```python
from build123d import *

# Parameters (mm, degrees)
ESQUISSE1_W             = 60
ESQUISSE1_H             = 60
ESQUISSE1_R             = 20
BOSS_EXTRU_1_DEPTH      = 25
CONG_1_R                = 1
TROU_TARAUD_M61_REACH   = 73.589
TROU_TARAUD_M61_BORE_R  = 2.5
TROU_TARAUD_M41_D       = 3.3
TROU_TARAUD_M41_DEPTH   = 7.5
TROU_TARAUD_M41_TIP     = 0.991420021
TROU_TARAUD_M42_D       = 3.3
TROU_TARAUD_M42_DEPTH   = 10.5
TROU_TARAUD_M42_TIP     = 0.991420021
ENL_V_MAT_EXTRU_1_REACH = 51.244
ENL_V_MAT_EXTRU_2_DEPTH = 3


with BuildPart() as part:
    # Esquisse1 → Boss.-Extru.1 (new body)
    with BuildSketch(Plane(origin=(0, 0, 0), x_dir=(1, 0, 0), z_dir=(0, 1, 0))):
        Rectangle(ESQUISSE1_W, ESQUISSE1_H)
        with Locations(Location((0, 0, 0), (0, 0, 270))):
            Circle(ESQUISSE1_R, mode=Mode.SUBTRACT)
    extrude(amount=BOSS_EXTRU_1_DEPTH)

    # Congé1
    cong_1_edges = [part.edges().sort_by_distance(p)[0] for p in [
        (30, 25, 0),
        (0, 25, -30),
        (-30, 25, 0),
        (0, 0, -30),
        (30, 0, 0),
        (0, 0, 30),
        (-30, 0, 0),
        (0, 25, 30),
        (-30, 12.5, -30),
        (30, 12.5, -30),
        (30, 12.5, 30),
        (-30, 12.5, 30),
    ]]
    fillet(cong_1_edges, radius=CONG_1_R)

    # Trou taraudé M61 bore → Trou taraudé M61 (cut, up to next)
    with BuildSketch(Plane.XY.offset(30), mode=Mode.PRIVATE) as trou_taraud_m61_sk1:
        with Locations((0, 12.5)):
            Circle(TROU_TARAUD_M61_BORE_R)
    trou_taraud_m61_tool1 = extrude(trou_taraud_m61_sk1.sketch, amount=-TROU_TARAUD_M61_REACH, mode=Mode.PRIVATE) & part.part
    add(trou_taraud_m61_tool1.solids().sort_by_distance((0, 12.5, 30))[0], mode=Mode.SUBTRACT)

    # Trou taraudé M41
    with Locations(Plane(origin=(0, 0, -30), x_dir=(-1, 0, 0), z_dir=(0, 0, -1))):
        with Locations((11.7, 12.5), (-11.7, 12.5)):
            Hole(TROU_TARAUD_M41_D / 2, depth=TROU_TARAUD_M41_DEPTH)
            with Locations((0, 0, -(TROU_TARAUD_M41_DEPTH + TROU_TARAUD_M41_TIP / 2))):  # 118° drill point
                Cone(0, TROU_TARAUD_M41_D / 2, TROU_TARAUD_M41_TIP, mode=Mode.SUBTRACT)

    # Trou taraudé M42
    with Locations(Plane.ZY.offset(30)):
        with Locations((-9.666666667, 12.5)):
            Hole(TROU_TARAUD_M42_D / 2, depth=TROU_TARAUD_M42_DEPTH)
            with Locations((0, 0, -(TROU_TARAUD_M42_DEPTH + TROU_TARAUD_M42_TIP / 2))):  # 118° drill point
                Cone(0, TROU_TARAUD_M42_D / 2, TROU_TARAUD_M42_TIP, mode=Mode.SUBTRACT)

    # Esquisse10 → Enlèv. mat.-Extru.1 (cut, up to next)
    with BuildSketch(Plane.XZ, mode=Mode.PRIVATE) as enl_v_mat_extru_1_sk1:
        with BuildLine():
            Line((-6, 19.078784028), (-6, 23.3))
            Line((-6, 23.3), (6, 23.3))
            Line((6, 23.3), (6, 19.078784028))
            ThreePointArc((6, 19.078784028), (0, 20), (-6, 19.078784028))
        make_face()
    enl_v_mat_extru_1_tool1 = extrude(enl_v_mat_extru_1_sk1.sketch, amount=-ENL_V_MAT_EXTRU_1_REACH, mode=Mode.PRIVATE) & part.part
    add(enl_v_mat_extru_1_tool1.solids().sort_by_distance((0, 0, 21.487514))[0], mode=Mode.SUBTRACT)

    # Esquisse11 → Enlèv. mat.-Extru.2 (cut)
    with BuildSketch(Plane.XZ):
        with BuildLine():
            Line((-10, 30), (-10, 17.320508076))
            ThreePointArc((-10, 17.320508076), (0, 20), (10, 17.320508076))
            Line((10, 17.320508076), (10, 30))
            Line((10, 30), (-10, 30))
        make_face()
    enl_v_mat_extru_2 = extrude(amount=-ENL_V_MAT_EXTRU_2_DEPTH, mode=Mode.SUBTRACT)

    # Esquisse13 → Trou taraudé M31 (revolve, cut)
    with BuildSketch(Plane(origin=(0, 3, 26), x_dir=(0, 0, -1), z_dir=(1, 0, 0))):
        Polygon((0, 0), (0, 6.251075774), (1.25, 5.5), (1.25, 0), align=None)
    trou_taraud_m31 = revolve(axis=Axis((0, -3.35, 26), (0, 1, 0)), mode=Mode.SUBTRACT)

    # Symétrie1: Enlèv. mat.-Extru.2, Trou taraudé M31 across plane
    add(enl_v_mat_extru_2.mirror(Plane(origin=(0, 12.5, 0), x_dir=(0, 0, 1), z_dir=(0, -1, 0))), mode=Mode.SUBTRACT)
    add(trou_taraud_m31.mirror(Plane(origin=(0, 12.5, 0), x_dir=(0, 0, 1), z_dir=(0, -1, 0))), mode=Mode.SUBTRACT)


solid = part.part
```
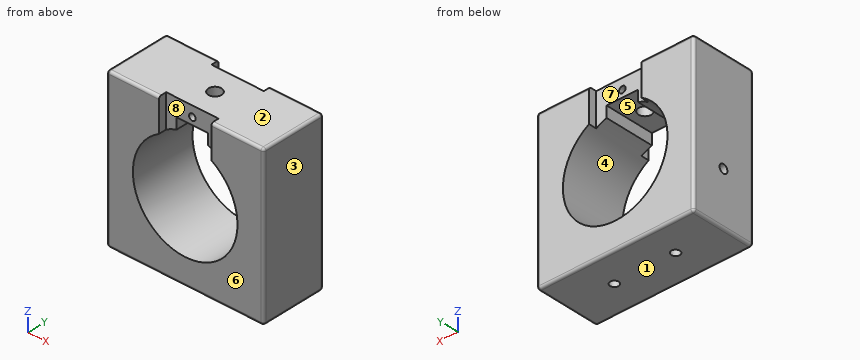
Model file for the job. Use its own axes, mm. Face numbers are marked on the shaded views. A direction names the side the tool comes from. Round coordinates to 2 decimals unless told otherwise and drop trailing zeros. Write each loop counter-clockwise with the first axis right and the second up, starting at its lowest first coordinate (ties: lowest second). Pieces come first, ordered by that corner, then holes. Notation, with made-up numbers: (6.5, 11.25) -> (61.5, 11.25) arc R22 ccw to (61.5, 44.25) -> close; hole circle Ø11 at (10.25, -35). An arc over 180 degrees is marked (long way). Answer as CSV lines item,"result".
1. Slice it at C-C, the plane x = -14.5. List the corners of the cut face in (y, z), plus the area to 3 significant figures.
Resolved:
outline,"(0, -29) arc R1 ccw to (1, -30) -> (24, -30) arc R1 ccw to (25, -29) -> (25, -13.77) -> (0, -13.77) -> close; (0, 13.77) -> (25, 13.77) -> (25, 29) arc R1 ccw to (24, 30) -> (1, 30) arc R1 ccw to (0, 29) -> close"
area,"810 mm²"
2. Tool access for the marked faces 5, 6, 7 and 8: list every direction of +Z, -Z, +X, -X, +Y, -Y with a clear straight run to the whole face (end or side of a thin tool).
Resolved:
face 5,"+Y, -Y"
face 6,"+Z, -Z, +X, -X, -Y"
face 7,"+Z, +Y"
face 8,"+Z, -Y"
3. Mould opens along Z. For the marked faces 1, 2, 3 and 4 say: +Z half, -Z half, draft (parallel to the pull), parting line (faces both ways), or undercut.
Resolved:
face 1,"-Z half"
face 2,"+Z half"
face 3,"draft"
face 4,"undercut"
4. Drill centre lines: line 1 (X direction, y = 12.5, z = -28.5); line 2 (X direction, y = 7.75, z = 23); line 3 (X direction, y = 18.6, z = 26). Where is each one in solid material? Low to high.
Resolved:
line 1,"-30 to -13.35, -10.05 to 10.05, 13.35 to 30"
line 2,"-30 to -6, 6 to 30"
line 3,"-30 to -1.25, 1.25 to 30"
5. Slice it at B-B, the plane y = 23.25. List the corners of the cut face in (x, z), plus the area to 3 significant figures.
Resolved:
outline,"(-30, -29) arc R1 ccw to (-29, -30) -> (29, -30) arc R1 ccw to (30, -29) -> (30, 29) arc R1 ccw to (29, 30) -> (10, 30) -> (10, 17.32) arc R20 cw (long way) to (-10, 17.32) -> (-10, 30) -> (-29, 30) arc R1 ccw to (-30, 29) -> close"
area,"2,130 mm²"
6. Slice it at A-A, the plane z = 0. List the corners of the cut face in (x, y).
Resolved:
outline,"(-30, 1) arc R1 ccw to (-29, 0) -> (-20, 0) -> (-20, 25) -> (-29, 25) arc R1 ccw to (-30, 24) -> close; (20, 0) -> (29, 0) arc R1 ccw to (30, 1) -> (30, 24) arc R1 ccw to (29, 25) -> (20, 25) -> close"
7. Pin check, flat tips, straight feed: pin 1 Ø6.5 at (x, z) = (1, 22) entering from -Y; pin 2 Ø2 at (x, z) = (0, 26) entering from +Y; pin 3 Ø2 at (x, z) = (0, 26) entering from -Y. Stop position of each tip, or through.
Resolved:
pin 1,"y = 3"
pin 2,"y = 16.35"
pin 3,"y = 8.65"
